For this review, take the finished solid that the model builds, in its own axes (mm). Give positions to 0.01 mm unless a question says otherwise; leave off trailing zeros. Loops run counter-clockwise (first coordinate to the right, second up) from the corner with the lowest first, then second, coordinate; pieces in that order, holes last. Notation, with made-up numbers: M 22.25,13 L 57.25,13 A33 ccw 57.25,42 Z; hole C 79.25,-38 d3. An arc over 180 degrees is marked long. Use CSV: the item, a comma, the result in double quotes. Start each with the question number.
1. The part is to be moulded in two halves that separate along Y. For faces 1 (the face through (37.2, 180.9, 2)), 2 (the face through (90, 74, 4)), say which applies: pulls with the +Y half, pulls with the -Y half, needs draft (parallel to the pull), parting line crosses it, or undercut.
2. Take a section at A-A, the plane y = 183. Write out the cut boundary in (x, z).
3. Insertion check: P1, Ø2, axis at x = 179.5, z = 1, coming from the +Y side; P2, Ø1.2, axis at x = -1.5, z = 2.5, coming from the -Y side; P3, Ø2, axis at x = 17.5, z = 3, coming from the -Y side. Each pin has a flat end and moves straight along its axis. Give the tip position at first contact, or say it passes through.
4. To check wall thickness, follow line 1 (Y direction, x = 80.5, z = 3.05); line 2 (Y direction, x = 40, z = 1.75); line 3 (Y direction, x = 49, z = 2.2). State the ranges of each line that lie inside material, in increasing order. Write a range as [from, to].
5. Take a section at B-B, the plane x = 144. Write out the cut boundary in (y, z).
6. Take a section at D-D, the plane y = 85. Write out the cut boundary in (x, z), and give its area (3 significant figures).
7. Take a section at C-C, the plane x = 40. Write out the cut boundary in (y, z), and give its area (3 significant figures).
from build123d import *

# Parameters (mm, degrees)
SKETCH_1_W      = 4.4
SKETCH_1_H      = 20.4
SKETCH_1_W_2    = 30.4
SKETCH_1_H_2    = 4.4
SKETCH_1_R      = 3.5
EXTRUDE_1_DEPTH = 4


with BuildPart() as part:
    # Эскиз1 → Бобышка-Вытянуть1 (new body)
    with BuildSketch(Plane.XY):
        Polygon((0, 20), (0, 0), (27, 0), (27, -4), (57, -4), (57, 0), (137, 0), (137, -4), (167, -4), (167, 0), (187, 0), (187, 133), (50, 133), (50, 193), (30, 193), (30, 133), (0, 133), (0, 120), (-4, 120), (-4, 100), (0, 100), (0, 40), (-4, 40), (-4, 20), align=None)
        with Locations((79, 35)):
            Rectangle(SKETCH_1_W, SKETCH_1_H, mode=Mode.SUBTRACT)
        with Locations((43.5, 67.2)):
            Rectangle(SKETCH_1_W_2, SKETCH_1_H_2, mode=Mode.SUBTRACT)
        with Locations((79, 80)):
            Rectangle(SKETCH_1_W, SKETCH_1_H, mode=Mode.SUBTRACT)
        with Locations((179, 35)):
            Rectangle(SKETCH_1_W, SKETCH_1_H, mode=Mode.SUBTRACT)
        with Locations((143.5, 67.2)):
            Rectangle(SKETCH_1_W_2, SKETCH_1_H_2, mode=Mode.SUBTRACT)
        with Locations((179, 80)):
            Rectangle(SKETCH_1_W, SKETCH_1_H, mode=Mode.SUBTRACT)
        with Locations((179, 113.3)):
            Rectangle(SKETCH_1_W, SKETCH_1_H, mode=Mode.SUBTRACT)
        with Locations((40, 183)):
            Circle(SKETCH_1_R, mode=Mode.SUBTRACT)
    extrude(amount=EXTRUDE_1_DEPTH)


solid = part.part
Result set:
1,face 1,"undercut"
1,face 2,"needs draft"
2,outline,"M 30,0 L 36.5,0 L 36.5,4 L 30,4 Z; M 43.5,0 L 50,0 L 50,4 L 43.5,4 Z"
3,P1,"y = 133"
3,P2,"y = 20"
3,P3,"y = 0"
4,line 1,"[0, 24.8], [45.2, 69.8], [90.2, 133]"
4,line 2,"[-4, 65], [69.4, 179.5], [186.5, 193]"
4,line 3,"[-4, 65], [69.4, 193]"
5,outline,"M -4,0 L 65,0 L 65,4 L -4,4 Z; M 69.4,0 L 133,0 L 133,4 L 69.4,4 Z"
6,outline,"M 0,0 L 76.8,0 L 76.8,4 L 0,4 Z; M 81.2,0 L 176.8,0 L 176.8,4 L 81.2,4 Z; M 181.2,0 L 187,0 L 187,4 L 181.2,4 Z"
6,area,"713 mm2"
7,outline,"M -4,0 L 65,0 L 65,4 L -4,4 Z; M 69.4,0 L 179.5,0 L 179.5,4 L 69.4,4 Z; M 186.5,0 L 193,0 L 193,4 L 186.5,4 Z"
7,area,"742 mm2"
